Check sheet for the modelled part. Datum: model origin and axes. Units: mm. Face numbers are marked on the shaded views. Round coordinates to 2 decimals unless told otherwise and drop trailing zeros. Loops run counter-clockwise (first coordinate to the right, second up) from the corner with the lowest first, then second, coordinate; pieces in that order, holes last. Notation, with made-up numbers: (73, 75) - (83, 75) arc R22 cw to (83, 114) - close; hole circle Ø1 at (86, 66). An arc over 180 degrees is marked (long way). Put each result on its own line as item: value. Start each with the question number.
Item 1: Section check A-A, the plane z = 60. Record the cut outline in (x, y).
Item 2: Gauge pin test, flat ends, axial feed: pin 1 Ø3 at (x, y) = (15.5, -0.5) entering from +Z; pin 2 Ø1 at (y, z) = (-1.5, 18) entering from -X; pin 3 Ø1.5 at (y, z) = (2.5, 44) entering from -X; pin 4 Ø16 at (x, z) = (-6.5, 29.5) entering from +Y. Record the tip position at first contact, or that the pin passes through.
Item 3: Draft check along X on the marked faces 1, 2 and 3. Enter one of: pulls with the +X half, pulls with the -X half, needs draft (parallel to the pull), parting line crosses it, or undercut.
Item 4: Material ranges on line 1 along X through (y, z) = (-1, 60); line 2 along Z through (x, y) = (0, -0.7); line 3 along Z through (x, y) = (17.5, 1.5), recorded low to high.
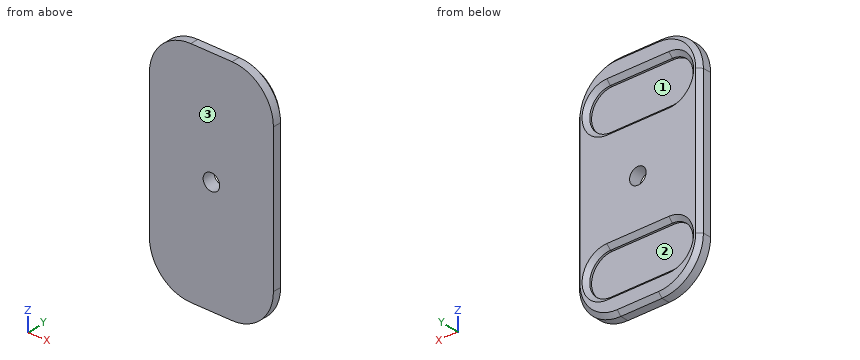
from build123d import *

# Parameters (mm, degrees)
SKETCH1_W           = 60
SKETCH1_H           = 70
BOSS_EXTRUDE1_DEPTH = 3
SKETCH2_W           = 60
SKETCH2_H           = 140
BOSS_EXTRUDE2_DEPTH = 3
SKETCH4_W           = 60
SKETCH4_H           = 5
CUT_EXTRUDE1_DEPTH  = 10
CHAMFER2_SIZE       = 15
SKETCH5_R           = 4
CUT_EXTRUDE2_DEPTH  = 3
FILLET3_R           = 20
CHAMFER3_SIZE       = 1
SKETCH6_W           = 103.197432935
SKETCH6_H           = 87.20183083
CUT_EXTRUDE3_DEPTH  = 100
SKETCH7_W           = 60
SKETCH7_H           = 55
BOSS_EXTRUDE3_DEPTH = 3
SKETCH8_W           = 60
SKETCH8_H           = 55
BOSS_EXTRUDE4_DEPTH = 3
FILLET4_R           = 20
CHAMFER4_SIZE       = 2
SKETCH9_R           = 4
CUT_EXTRUDE4_DEPTH  = 10


with BuildPart() as part:
    # Sketch1 → Boss-Extrude1 (new body)
    with BuildSketch(Plane(origin=(0, 0, 0), x_dir=(1, 0, 0), z_dir=(0, 1, 0))):
        with Locations((0, -35)):
            Rectangle(SKETCH1_W, SKETCH1_H)
        with BuildLine():
            Line((-15, -35), (15, -35))
            ThreePointArc((15, -35), (25, -25), (15, -15))
            Line((15, -15), (-15, -15))
            ThreePointArc((-15, -15), (-25, -25), (-15, -35))
        make_face(mode=Mode.SUBTRACT)
    boss_extrude1 = extrude(amount=BOSS_EXTRUDE1_DEPTH)

    # Mirror1: Boss-Extrude1 across plane
    add(boss_extrude1.mirror(Plane(origin=(-30, 3, 70), x_dir=(1, 0, 0), z_dir=(0, 0, -1))))

    # Sketch2 → Boss-Extrude2 (add)
    with BuildSketch(Plane(origin=(0, 0, 0), x_dir=(-1, 0, 0), z_dir=(0, -1, 0))):
        with Locations((0, -70)):
            Rectangle(SKETCH2_W, SKETCH2_H)
    boss_extrude2 = extrude(amount=BOSS_EXTRUDE2_DEPTH)

    # Sketch4 → Cut-Extrude1 (cut)
    with BuildSketch(Plane(origin=(0, 3, 0), x_dir=(1, 0, 0), z_dir=(0, 1, 0))):
        with Locations((0, -2.5)):
            Rectangle(SKETCH4_W, SKETCH4_H)
        with Locations((0, -137.5)):
            Rectangle(SKETCH4_W, SKETCH4_H)
    cut_extrude1 = extrude(amount=-CUT_EXTRUDE1_DEPTH, mode=Mode.SUBTRACT)

    # Chamfer2
    chamfer2_edges = [part.edges().sort_by_distance(p)[0] for p in [
        (30, 0, 5),
        (-30, 0, 5),
        (30, 0, 135),
        (-30, 0, 135),
    ]]
    chamfer(chamfer2_edges, length=CHAMFER2_SIZE)

    # Sketch5 → Cut-Extrude2 (cut)
    with BuildSketch(Plane.XZ.offset(3)):
        with Locations((0, 70)):
            Circle(SKETCH5_R)
    extrude(amount=-CUT_EXTRUDE2_DEPTH, mode=Mode.SUBTRACT)

    # Fillet3
    fillet3_edges = [part.edges().sort_by_distance(p)[0] for p in [
        (-30, 0, 20),
        (-30, 0, 120),
        (15, 0, 135),
        (-15, 0, 135),
        (30, 0, 20),
        (30, 0, 120),
        (-15, 0, 5),
        (15, 0, 5),
    ]]
    fillet(fillet3_edges, radius=FILLET3_R)

    # Chamfer3
    chamfer3_edges = [part.edges().sort_by_distance(p)[0] for p in [
        (25, 3, 25),
        (0, 3, 15),
        (-25, 3, 25),
        (0, 3, 35),
        (30, 3, 70),
        (-30, 3, 70),
        (-22.5, 3, 127.5),
        (0, 3, 135),
        (22.5, 3, 127.5),
        (22.5, 3, 12.5),
        (0, 3, 5),
        (-22.5, 3, 12.5),
        (-14.3693974, 3, 133.47759065),
        (-28.47759065, 3, 119.3693974),
        (14.3693974, 3, 133.47759065),
        (28.47759065, 3, 119.3693974),
        (-28.47759065, 3, 20.6306026),
        (-14.3693974, 3, 6.52240935),
        (14.3693974, 3, 6.52240935),
        (28.47759065, 3, 20.6306026),
        (25, 3, 115),
        (0, 3, 125),
        (-25, 3, 115),
        (0, 3, 105),
    ]]
    chamfer(chamfer3_edges, length=CHAMFER3_SIZE)

    # Sketch6 → Cut-Extrude3 (cut)
    with BuildSketch(Plane(origin=(0, 3, 0), x_dir=(1, 0, 0), z_dir=(0, 1, 0))):
        with Locations((0.064498395, -103.600915415)):
            Rectangle(SKETCH6_W, SKETCH6_H)
    cut_extrude3 = extrude(amount=-CUT_EXTRUDE3_DEPTH, mode=Mode.SUBTRACT)

    # Mirror4: Boss-Extrude1, Boss-Extrude2, Cut-Extrude1, Cut-Extrude3 across plane
    add(boss_extrude1.mirror(Plane(origin=(-51.534218072, -97, 60), x_dir=(1, 0, 0), z_dir=(0, 0, -1))))
    add(boss_extrude2.mirror(Plane(origin=(-51.534218072, -97, 60), x_dir=(1, 0, 0), z_dir=(0, 0, -1))))
    add(cut_extrude1.mirror(Plane(origin=(-51.534218072, -97, 60), x_dir=(1, 0, 0), z_dir=(0, 0, -1))), mode=Mode.SUBTRACT)
    add(cut_extrude3.mirror(Plane(origin=(-51.534218072, -97, 60), x_dir=(1, 0, 0), z_dir=(0, 0, -1))), mode=Mode.SUBTRACT)

    # Sketch7 → Boss-Extrude3 (add)
    with BuildSketch(Plane(origin=(0, 3, 0), x_dir=(1, 0, 0), z_dir=(0, 1, 0))):
        with Locations((0, -32.5)):
            Rectangle(SKETCH7_W, SKETCH7_H)
        with BuildLine():
            Line((-15, -35), (15, -35))
            ThreePointArc((15, -35), (25, -25), (15, -15))
            Line((15, -15), (-15, -15))
            ThreePointArc((-15, -15), (-25, -25), (-15, -35))
        make_face(mode=Mode.SUBTRACT)
    extrude(amount=-BOSS_EXTRUDE3_DEPTH)

    # Sketch8 → Boss-Extrude4 (add)
    with BuildSketch(Plane(origin=(0, 0, 0), x_dir=(-1, 0, 0), z_dir=(0, -1, 0))):
        with Locations((0, -32.5)):
            Rectangle(SKETCH8_W, SKETCH8_H)
    extrude(amount=BOSS_EXTRUDE4_DEPTH)

    # Fillet4
    fillet4_edges = [part.edges().sort_by_distance(p)[0] for p in [
        (30, 0, 115),
        (-30, 0, 115),
        (-30, 0, 5),
        (30, 0, 5),
    ]]
    fillet(fillet4_edges, radius=FILLET4_R)

    # Chamfer4
    chamfer4_edges = [part.edges().sort_by_distance(p)[0] for p in [
        (25, 3, 95),
        (0, 3, 105),
        (-25, 3, 95),
        (0, 3, 85),
        (-25, 3, 25),
        (0, 3, 15),
        (25, 3, 25),
        (0, 3, 35),
        (0, 3, 115),
        (30, 3, 60),
        (0, 3, 5),
        (-30, 3, 60),
        (-24.142135624, 3, 10.857864376),
        (24.142135624, 3, 10.857864376),
        (-24.142135624, 3, 109.142135624),
        (24.142135624, 3, 109.142135624),
    ]]
    chamfer(chamfer4_edges, length=CHAMFER4_SIZE)

    # Sketch9 → Cut-Extrude4 (cut)
    with BuildSketch(Plane(origin=(0, -3, 0), x_dir=(-1, 0, 0), z_dir=(0, -1, 0))):
        with Locations((0, -60)):
            Circle(SKETCH9_R)
    extrude(amount=-CUT_EXTRUDE4_DEPTH, mode=Mode.SUBTRACT)


solid = part.part
Check result:
1. outline: (-30, -3) - (-4, -3) - (-4, 3) - (-28, 3) - (-30, 1) - close; (4, -3) - (30, -3) - (30, 1) - (28, 3) - (4, 3) - close
2. pin 1: z = 114.6
2. pin 2: x = -28.91
2. pin 3: x = -29.25
2. pin 4: y = 3
3. face 1: undercut
3. face 2: undercut
3. face 3: needs draft
4. line 1: -30 to -4, 4 to 30
4. line 2: 5 to 56, 64 to 115
4. line 3: 7 to 14.8, 35.2 to 84.8, 105.2 to 113
